Geometry: final body of the model. Coordinates: model frame, mm. A direction names the side the tool comes from. Coordinates: 2 decimals unless noted, no trailing zeros. Write each loop counter-clockwise with the first axis right and the second up, starting at its lowest first coordinate (ties: lowest second). Pieces come first, ordered by that corner, then holes. Notation, with made-up numbers: (11, -9.5) -> (15, -9.5) arc R12 ccw to (15, -0.5) -> close; hole circle Ø11 at (-2.75, -15). An arc over 180 degrees is marked (long way). One line per item, written item: value.
```python
from build123d import *

# Parameters (mm, degrees)
F1_DEPTH = 29
F2_W     = 5.75
F2_H     = 23
F3_DEPTH = 4
F2_W_2   = 3.5
F2_H_2   = 4
F4_DEPTH = 4.001


with BuildPart() as f1:
    # F0 (on Front) → F1 (new body)
    with BuildSketch(Plane.XZ):
        Polygon((0, 4), (0, 0), (50.75, 0), (50.75, 3.25), (50.75, 4), (50.15, 4), (50.15, 3.25), (48.744, 3.25), (48.744, 4), (48.144, 4), (48.144, 3.25), (46.738, 3.25), (46.738, 4), (46.138, 4), (46.138, 3.25), (44.732, 3.25), (44.732, 4), (44.132, 4), (44.132, 3.25), (42.726, 3.25), (42.726, 4), (42.126, 4), (42.126, 3.25), (40.72, 3.25), (40.72, 4), (40.12, 4), (40.12, 3.25), (38.714, 3.25), (38.714, 4), (38.114, 4), (38.114, 3.25), (36.708, 3.25), (36.708, 4), (36.108, 4), (36.108, 3.25), (34.702, 3.25), (34.702, 4), (34.102, 4), (34.102, 3.25), (32.696, 3.25), (32.696, 4), (32.096, 4), (32.096, 3.25), (30.69, 3.25), (30.69, 4), (30.09, 4), (30.09, 3.25), (28.684, 3.25), (28.684, 4), (28.084, 4), (28.084, 3.25), (26.678, 3.25), (26.678, 4), (26.078, 4), (26.078, 3.25), (24.672, 3.25), (24.672, 4), (24.072, 4), (24.072, 3.25), (22.666, 3.25), (22.666, 4), (22.066, 4), (22.066, 3.25), (20.66, 3.25), (20.66, 4), (20.06, 4), (20.06, 3.25), (18.654, 3.25), (18.654, 4), (18.054, 4), (18.054, 3.25), (16.648, 3.25), (16.648, 4), (16.048, 4), (16.048, 3.25), (14.642, 3.25), (14.642, 4), (14.042, 4), (14.042, 3.25), (12.636, 3.25), (12.636, 4), (12.036, 4), (12.036, 3.25), (10.63, 3.25), (10.63, 4), (10.03, 4), (10.03, 3.25), (8.624, 3.25), (8.624, 4), (8.324, 4), (8.024, 4), (8.024, 3.25), (6.618, 3.25), (6.618, 4), (6.318, 4), (6.018, 4), (6.018, 3.25), (4.612, 3.25), (4.612, 4), (4.012, 4), (4.012, 3.25), (2.606, 3.25), (2.606, 4), (2.006, 4), (2.006, 3.25), (0.6, 3.25), (0.6, 4), align=None)
    extrude(amount=F1_DEPTH)

    # F2 (on face) → F3 (cut, through all)
    with BuildSketch(Plane(origin=(0, 0, 0), x_dir=(1, 0, 0), z_dir=(0, 0, -1))):
        with Locations((22.5, 17.5)):
            Rectangle(F2_W, F2_H)
        with Locations((28.25, 17.5)):
            Rectangle(F2_W, F2_H)
    extrude(amount=-F3_DEPTH, mode=Mode.SUBTRACT)

    # F2 (on face) → F4 (cut, through all)
    with BuildSketch(Plane(origin=(0, 0, 0), x_dir=(1, 0, 0), z_dir=(0, 0, -1))):
        with BuildLine():
            ThreePointArc((12.625, 23), (10.875, 24.75), (9.125, 23))
            Line((9.125, 23), (12.625, 23))
        make_face()
        with Locations((10.875, 21)):
            Rectangle(F2_W_2, F2_H_2)
        with BuildLine():
            Line((12.625, 19), (9.125, 19))
            ThreePointArc((9.125, 19), (10.875, 17.25), (12.625, 19))
        make_face()
        with BuildLine():
            ThreePointArc((12.625, 8.75), (10.875, 10.5), (9.125, 8.75))
            Line((9.125, 8.75), (12.625, 8.75))
        make_face()
        with Locations((10.875, 6.75)):
            Rectangle(F2_W_2, F2_H_2)
        with BuildLine():
            Line((12.625, 4.75), (9.125, 4.75))
            ThreePointArc((9.125, 4.75), (10.875, 3), (12.625, 4.75))
        make_face()
        with BuildLine():
            ThreePointArc((41.5842387676, 23), (39.8342387676, 24.75), (38.0842387676, 23))
            Line((38.0842387676, 23), (41.5842387676, 23))
        make_face()
        with Locations((39.8342387676, 21)):
            Rectangle(F2_W_2, F2_H_2)
        with BuildLine():
            Line((41.5842387676, 19), (38.0842387676, 19))
            ThreePointArc((38.0842387676, 19), (39.8342387676, 17.25), (41.5842387676, 19))
        make_face()
        with BuildLine():
            ThreePointArc((41.625, 8.75), (39.875, 10.5), (38.125, 8.75))
            Line((38.125, 8.75), (41.625, 8.75))
        make_face()
        with Locations((39.875, 6.75)):
            Rectangle(F2_W_2, F2_H_2)
        with BuildLine():
            Line((41.625, 4.75), (38.125, 4.75))
            ThreePointArc((38.125, 4.75), (39.875, 3), (41.625, 4.75))
        make_face()
    extrude(amount=-F4_DEPTH, mode=Mode.SUBTRACT)


solid = f1.part
```
(1) Line query: line 1 (X direction, y = -4.75, z = 1.5) (3 decimals); line 2 (X direction, y = -20.5, z = 0.2) (3 decimals); line 3 (X direction, y = -17.5, z = 1.1) (3 decimals). Output: solid intervals per line, ascending. Write a range as [from, to].
Responses:
line 1: x = [0, 9.125], [12.625, 38.125], [41.625, 50.75]
line 2: x = [0, 9.125], [12.625, 19.625], [31.125, 38.084], [41.584, 50.75]
line 3: x = [0, 9.974], [11.776, 19.625], [31.125, 38.933], [40.736, 50.75]
(2) Section A-A (z = 2.5). Return the cut outline in (x, y) (3 decimals), then the cut area to 3 significant figures.
Responses:
outline: (0, -29) -> (19.625, -29) -> (19.625, -6) -> (31.125, -6) -> (31.125, -29) -> (50.75, -29) -> (50.75, 0) -> (0, 0) -> close; hole (9.125, -23) arc R1.75 ccw to (12.625, -23) -> (12.625, -19) arc R1.75 ccw to (9.125, -19) -> close; hole (9.125, -8.75) arc R1.75 ccw to (12.625, -8.75) -> (12.625, -4.75) arc R1.75 ccw to (9.125, -4.75) -> close; hole (38.084, -23) arc R1.75 ccw to (41.584, -23) -> (41.584, -19) arc R1.75 ccw to (38.084, -19) -> close; hole (38.125, -8.75) arc R1.75 ccw to (41.625, -8.75) -> (41.625, -4.75) arc R1.75 ccw to (38.125, -4.75) -> close
area: 1,110 mm2
(3) Pull-direction query (X, two-part tool) for faces 4 (the flat face through (25, 0, 2)), 5 (the flat face through (39, -14, 3.25)); classes: released by +X, released by -X, zero draft, split by the parting line, or undercut.
Responses:
face 4: zero draft
face 5: undercut
(4) First-contact query: pin 1 (0.7 mm diameter, centred on x = 5.5, y = -14.5, fed in from +Z). Flat tip, straight axial feed; report the tip coordinate or a pass-through.
Responses:
pin 1: stops at z = 3.25
(5) Section B-B (y = -6.5). State how many separate pieces and enclosed holes the cut face has, then the cut area to 3 significant figures.
Responses:
separate pieces: 4
enclosed holes: 0
area: 112 mm2
(6) Reachability of faces 1 (the flat face through (11, -27, 3.25)), 2 (the cylindrical face through (39.8, -3, 1.5)), 3 (the flat face through (31.125, -17, 2)) from +Z, -Z, +X, -X, +Y, -Y: full face, straight path, thin tool, end or side. Return the list, or none.
Responses:
face 1: +Z, +Y, -Y
face 2: +Z, -Z
face 3: +Z, -Z, -Y
